Build history of the part. All positions in model axes, mm. A direction names the side the tool comes from. Round coordinates to 2 decimals unless told otherwise and drop trailing zeros. Order: outer loops, then holes, each group sorted by start corner. A loop starts at its lowest first (then second) coordinate and runs counter-clockwise, first axis right, second up. Notation, with made-up numbers: M 47.5,-11.5 L 74.5,-11.5 A14 ccw 74.5,-7.5 Z; hole C -33,54.25 d6. An arc over 180 degrees is marked long. One line per item, written item: value. Start each with the question number.
Item 1: Band-saw the part on B-B, the plane y = -7.25. Write the cut outline in (x, z), then the cut area to 3 significant figures.
Item 2: Band-saw the part on C-C, the plane x = -3.25. Write the cut outline in (y, z) (3 decimals), then the cut area to 3 significant figures.
Item 3: Band-saw the part on A-A, the plane x = -0.5. Write the cut outline in (y, z) (3 decimals).
Item 4: Pin check, flat tips, straight feed: pin 1 (2 mm diameter, centred on x = 3, y = -2, fed in from -Z); pin 2 (4 mm diameter, centred on y = -0.5, z = 1, fed in from +X). Stop position of each tip, or through.
Item 5: Tool access for faces 1 (the flat face through (-3.636, -1, 2)), 2 (the cylindrical face through (4.483, 6.76, 6.902)): list every direction of +Z, -Z, +X, -X, +Y, -Y with a clear straight run to the whole face (end or side of a thin tool).
Item 6: Band-saw the part on D-D, the plane y = 8.5. Write the cut outline in (x, z).
Item 7: Probe L1, parallel to X at y = 7.75, z = 10.75; L2, parallel to Y at x = 0, z = 3.75 (3 decimals); L3, parallel to Y at x = -0.5, z = 7.5 (3 decimals). List the from-to ranges inside material, lowest first.
Item 8: Two-plate mould, pull along Y, no slides. Class faces 3 (the flat face through (0, -10.875, 7)), 4 (the flat face through (-6.25, 0, 7)), 5 (the cylindrical face through (0.369, -9.525, 6.902)): +Y half, -Y half, draft (parallel to the pull), parting line (faces both ways), or undercut.
```python
from build123d import *

# Parameters (mm, degrees)
ESQUISSE1_W             = 12.5
ESQUISSE1_H             = 21.75
BOSS_EXTRU_3_DEPTH      = 14
ESQUISSE9_W             = 10.579409941
ESQUISSE9_H             = 6.787962443
ENL_V_MAT_EXTRU_7_DEPTH = 3.5
D_GAGEMENT_M32_D        = 3.4
D_GAGEMENT_M33_D        = 3.4
ESQUISSE23_W            = 9.88556754
ESQUISSE23_H            = 6.787962443
ESQUISSE23_R            = 1.7
BOSS_EXTRU_4_DEPTH      = 3.5


with BuildPart() as part:
    # Esquisse1 → Boss.-Extru.3 (new body)
    with BuildSketch(Plane.XY):
        Rectangle(ESQUISSE1_W, ESQUISSE1_H)
    extrude(amount=BOSS_EXTRU_3_DEPTH)

    # Esquisse9 → Enlèv. mat.-Extru.7 (cut)
    with BuildSketch(Plane.XY.offset(14)):
        with Locations((1.654137431, -1.292305661)):
            Rectangle(ESQUISSE9_W, ESQUISSE9_H)
    enl_v_mat_extru_7 = extrude(amount=-ENL_V_MAT_EXTRU_7_DEPTH, mode=Mode.SUBTRACT)

    # Dégagement M32 (through all)
    with Locations(Plane.XY.offset(14)):
        with Locations((-0.35, -1.306160818)):
            Hole(D_GAGEMENT_M32_D / 2)

    # Dégagement M33 (through all)
    with Locations(Plane.XY.offset(14)):
        with Locations((-3.63556754, 7.794867284), (3.134168266, 7.794867284), (0, -7.865811289)):
            Hole(D_GAGEMENT_M33_D / 2)

    # Symétrie1: Enlèv. mat.-Extru.7 across plane
    add(enl_v_mat_extru_7.mirror(Plane.XY.offset(7)), mode=Mode.SUBTRACT)

    # Esquisse23 → Boss.-Extru.4 (add)
    with BuildSketch(Plane.XY.offset(10.5)):
        with Locations((1.30721623, -1.292305661)):
            Rectangle(ESQUISSE23_W, ESQUISSE23_H)
        with Locations(Location((-0.35, -1.306160818, 0), (0, 0, 180))):
            Circle(ESQUISSE23_R, mode=Mode.SUBTRACT)
    extrude(amount=BOSS_EXTRU_4_DEPTH)


solid = part.part
```
Output:
1. outline: M -6.25,0 L -1.58,0 L -1.58,14 L -6.25,14 Z; M 1.58,0 L 6.25,0 L 6.25,14 L 1.58,14 Z
1. area: 131 mm²
2. outline: M -10.875,0 L -4.686,0 L -4.686,3.5 L 2.102,3.5 L 2.102,0 L 6.139,0 L 6.139,14 L -10.875,14 Z; M 9.451,0 L 10.875,0 L 10.875,14 L 9.451,14 Z
2. area: 234 mm²
3. outline: M -10.875,0 L -9.491,0 L -9.491,14 L -10.875,14 Z; M -6.241,0 L -4.686,0 L -4.686,3.5 L -3,3.5 L -3,14 L -6.241,14 Z; M 0.387,3.5 L 2.102,3.5 L 2.102,0 L 10.875,0 L 10.875,14 L 0.387,14 Z
4. pin 1: stops at z = 3.5
4. pin 2: stops at x = -3.64
5. face 1: -Z, +X
5. face 2: +Z, -Z
6. outline: M -6.25,0 L -5.18,0 L -5.18,14 L -6.25,14 Z; M -2.09,0 L 1.59,0 L 1.59,14 L -2.09,14 Z; M 4.68,0 L 6.25,0 L 6.25,14 L 4.68,14 Z
7. L1: x = -6.25 to -5.33, -1.94 to 1.43, 4.83 to 6.25
7. L2: y = -10.875 to -9.566, -6.166 to -2.97, 0.357 to 10.875
7. L3: y = -10.875 to -9.491, -6.241 to -3, 0.387 to 10.875
8. face 3: -Y half
8. face 4: draft
8. face 5: undercut
